```python
from build123d import *

# Parameters (mm, degrees)
F2_R     = 20
F3_DEPTH = 507.706612
F4_DEPTH = 346.473515


with BuildPart() as f1:
    # F0 (on Front) → F1 (revolve)
    with BuildSketch(Plane.XZ):
        Polygon((-122.14937, -25), (-26.473614, -25), (109.813852, -25), (109.813852, 0), (0, 0), (-26.473614, 0), (-122.14937, 0), align=None)
    revolve(axis=Axis((-122.14937, 0, 176.894253), (0, 0, 1)))

    # F2 (on face) → F3 (cut)
    with BuildSketch(Plane(origin=(0, 0, -25), x_dir=(1, 0, 0), z_dir=(0, 0, -1))):
        with Locations((-296.138028, 0)):
            Circle(F2_R)
    extrude(amount=-F3_DEPTH, mode=Mode.SUBTRACT)

    # F2 (on face) → F4 (cut)
    with BuildSketch(Plane(origin=(0, 0, -25), x_dir=(1, 0, 0), z_dir=(0, 0, -1))):
        with Locations((-249.620262, 118.417841)):
            Circle(F2_R)
        with Locations((-296.138028, 0)):
            Circle(F2_R)
        with BuildLine():
            ThreePointArc((-229.275148, -137.103469), (-225.584149, -130.955878), (-224.298739, -123.901511))
            ThreePointArc((-224.298739, -123.901511), (-263.01333, -116.847144), (-229.275148, -137.103469))
        make_face()
        with BuildLine():
            ThreePointArc((-102.14937, 173.988658), (-136.306099, 188.116185), (-122.108072, 153.9887))
            ThreePointArc((-122.108072, 153.9887), (-107.992641, 159.861131), (-102.14937, 173.988658))
        make_face()
        with BuildLine():
            ThreePointArc((21.757231, -122.144211), (-5.454588, -103.48973), (-13.041736, -135.597485))
            ThreePointArc((-13.041736, -135.597485), (8.96905, -140.798692), (21.757231, -122.144211))
        make_face()
        with BuildLine():
            ThreePointArc((-122.112818, -154.017654), (-135.839579, -159.476481), (-142.075022, -172.868345))
            ThreePointArc((-142.075022, -172.868345), (-132.108072, -173.730088), (-122.108072, -174.017653))
            Line((-122.108072, -174.017653), (-122.112818, -154.017654))
        make_face()
        with BuildLine():
            ThreePointArc((-122.108072, -174.017653), (-132.108072, -173.730088), (-142.075022, -172.868345))
            ThreePointArc((-142.075022, -172.868345), (-122.682964, -194.009389), (-102.108072, -174.017653))
            ThreePointArc((-102.108072, -174.017653), (-102.116336, -173.442761), (-102.141122, -172.868345))
            ThreePointArc((-102.141122, -172.868345), (-112.108072, -173.730088), (-122.108072, -174.017653))
        make_face()
        with BuildLine():
            ThreePointArc((-102.141122, -172.868345), (-108.380016, -159.473222), (-122.112818, -154.017654))
            Line((-122.112818, -154.017654), (-122.108072, -174.017653))
            ThreePointArc((-122.108072, -174.017653), (-112.108072, -173.730088), (-102.141122, -172.868345))
        make_face()
        with Locations((51.839288, 0)):
            Circle(F2_R)
        with Locations((0, 123.901511)):
            Circle(F2_R)
    extrude(amount=-F4_DEPTH, mode=Mode.SUBTRACT)


solid = f1.part
```
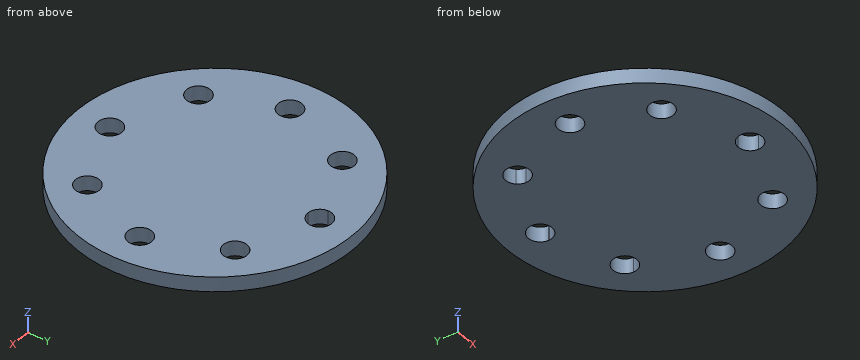
Input: part model. Units: mm. Frame: model coordinates. Give positions to 0.01 mm unless a question says otherwise; leave off trailing zeros. Order: outer loops, then holes, each group sorted by start corner. A loop starts at its lowest first (then second) coordinate and runs counter-clockwise, first axis right, second up. Notation, with made-up numbers: M -2.5,86.5 L 55.5,86.5 A11 ccw 55.5,104.5 Z; hole C 37,30 d8. An arc over 180 degrees is marked long. One line per question, with ' | ' between items.
1) Section A-A on y = 0. Output: boundary loops of the cut face in (x, z), and give its area (3 significant figures).
Filled in:
outline: M -354.11,-25 L -316.14,-25 L -316.14,0 L -354.11,0 Z; M -276.14,-25 L 31.84,-25 L 31.84,0 L -276.14,0 Z; M 71.84,-25 L 109.81,-25 L 109.81,0 L 71.84,0 Z | area: 9,600 mm2
2) Ray query, L1, parallel to Y at x = -245, z = -2.5; L2, parallel to Y at x = -131.5, z = -6.5; L3, parallel to Y at x = 60, z = -4.75. Return the intervals inside material, ascending.
Filled in:
L1: y = -196.76 to -137.88, -98.96 to 103.91, 143.89 to 196.76 | L2: y = -231.77 to -191.67, -156.31 to 156.36, 191.68 to 231.77 | L3: y = -143.63 to -18.26, 18.26 to 143.63
3) Contact query for flat-ended pins moving along their axis: P1, Ø12, axis at y = -169, z = -8.5, coming from the -X side; P2, Ø5, axis at y = 47, z = -8.5, coming from the +X side; P3, Ø4, axis at y = -162, z = -12, coming from the +X side; P4, Ø2, axis at x = -98, y = 89.5, coming from the +Z side. Output: stop coordinate, or through.
Filled in:
P1: stops at x = -287.19 | P2: stops at x = 105.51 | P3: stops at x = 45.8 | P4: stops at z = 0
4) Section D-D on y = 165.5. Output: boundary loops of the cut face in (x, z), and give its area (3 significant figures).
Filled in:
outline: M -284.68,-25 L -140.2,-25 L -140.2,0 L -284.68,0 Z; M -104.01,-25 L 40.38,-25 L 40.38,0 L -104.01,0 Z | area: 7,220 mm2
5) Section C-C on z = -19. State how many separate pieces and enclosed holes the cut face has, and give its area (3 significant figures).
Filled in:
separate pieces: 1 | enclosed holes: 8 | area: 159,000 mm2
6) Section B-B on x = 0. Output: boundary loops of the cut face in (y, z), and give its area (3 significant figures).
Filled in:
outline: M -197.2,-25 L -143.9,-25 L -143.9,0 L -197.2,0 Z; M -103.9,-25 L 102.22,-25 L 102.22,0 L -103.9,0 Z; M 142.07,-25 L 197.2,-25 L 197.2,0 L 142.07,0 Z | area: 7,860 mm2
